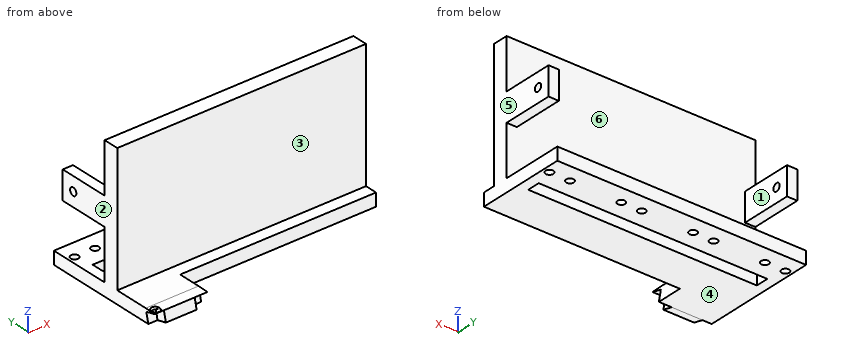
```python
from build123d import *

# Parameters (mm, degrees)
SKETCH1_W                      = 97
SKETCH1_H                      = 30
SKETCH1_R                      = 1.5
BOSS_EXTRUDE1_DEPTH            = 5
SKETCH2_W                      = 20.6
SKETCH2_H                      = 5
BOSS_EXTRUDE2_DEPTH            = 10
CUT_EXTRUDE1_REACH             = 99
CUT_EXTRUDE1_DIRECTION_2_DEPTH = 1
BOSS_EXTRUDE3_DEPTH            = 20.6
SKETCH5_W                      = 12
SKETCH5_H                      = 3.995489472
BOSS_EXTRUDE4_DEPTH            = 4.086588
SKETCH6_R                      = 1.6
CUT_EXTRUDE3_DEPTH             = 2
SKETCH7_W                      = 97
SKETCH7_H                      = 5
BOSS_EXTRUDE5_DEPTH            = 5
SKETCH8_W                      = 89.150949319
SKETCH8_H                      = 5
CUT_EXTRUDE5_DEPTH             = 6
SKETCH10_W                     = 97
SKETCH10_H                     = 6
BOSS_EXTRUDE7_DEPTH            = 50
SKETCH11_W                     = 4
SKETCH11_H                     = 11
BOSS_EXTRUDE8_DEPTH            = 20
SKETCH12_R                     = 1.5
CUT_EXTRUDE6_DEPTH             = 98


with BuildPart() as part:
    # Sketch1 → Boss-Extrude1 (new body)
    with BuildSketch(Plane.XY):
        Rectangle(SKETCH1_W, SKETCH1_H)
        with Locations((-46, 13.2)):
            Circle(SKETCH1_R, mode=Mode.SUBTRACT)
        with Locations((-38, 13.2)):
            Circle(SKETCH1_R, mode=Mode.SUBTRACT)
        with Locations((-18, 13.2)):
            Circle(SKETCH1_R, mode=Mode.SUBTRACT)
        with Locations((-10, 13.2)):
            Circle(SKETCH1_R, mode=Mode.SUBTRACT)
        with Locations((10, 13.2)):
            Circle(SKETCH1_R, mode=Mode.SUBTRACT)
        with Locations((18, 13.2)):
            Circle(SKETCH1_R, mode=Mode.SUBTRACT)
        with Locations((38, 13.2)):
            Circle(SKETCH1_R, mode=Mode.SUBTRACT)
        with Locations((46, 13.2)):
            Circle(SKETCH1_R, mode=Mode.SUBTRACT)
    extrude(amount=-BOSS_EXTRUDE1_DEPTH)

    # Sketch2 → Boss-Extrude2 (add)
    with BuildSketch(Plane.XZ.offset(15)):
        with Locations((-38.2, -2.5)):
            Rectangle(SKETCH2_W, SKETCH2_H)
    extrude(amount=BOSS_EXTRUDE2_DEPTH)

    # Sketch3 → Cut-Extrude1 (cut, up to next)
    with BuildSketch(Plane.ZY.offset(48.5), mode=Mode.PRIVATE) as cut_extrude1_sk1:
        Polygon((0, -25), (-5, -25), (0, -23.785067119), align=None)
    cut_extrude1_tool1 = extrude(cut_extrude1_sk1.sketch, amount=-CUT_EXTRUDE1_REACH, mode=Mode.PRIVATE) & part.part
    add(cut_extrude1_tool1.solids().sort_by_distance((-48.5, -24.595022, -1.666667))[0], mode=Mode.SUBTRACT)

    # Sketch3 → Cut-Extrude1 direction 2 (cut)
    with BuildSketch(Plane.ZY.offset(48.5)):
        Polygon((0, -25), (-5, -25), (0, -23.785067119), align=None)
    extrude(amount=CUT_EXTRUDE1_DIRECTION_2_DEPTH, mode=Mode.SUBTRACT)

    # Sketch4 → Boss-Extrude3 (add)
    with BuildSketch(Plane.ZY.offset(48.5)):
        Polygon((0, -23.785067119), (-1.117483581, -24.056600628), (-0.16158282, -27.990565936), align=None)
    extrude(amount=-BOSS_EXTRUDE3_DEPTH)

    # Sketch5 → Boss-Extrude4 (add)
    with BuildSketch(Plane(origin=(0, -22.459030354, 5.45724289), x_dir=(1, 0, 0), z_dir=(0, -0.971724853, 0.236116095))):
        with Locations((-38.9, -8.763781903)):
            Rectangle(SKETCH5_W, SKETCH5_H)
    extrude(amount=BOSS_EXTRUDE4_DEPTH)

    # Sketch6 → Cut-Extrude3 (cut)
    with BuildSketch(Plane(origin=(0, -1.597570275, -6.574726471), x_dir=(-1, 0, 0), z_dir=(0, -0.236116095, -0.971724853))):
        with Locations((46.634175133, -25.412540847)):
            Circle(SKETCH6_R)
    extrude(amount=-CUT_EXTRUDE3_DEPTH, mode=Mode.SUBTRACT)

    # Sketch7 → Boss-Extrude5 (add, through all)
    with BuildSketch(Plane.XY):
        with Locations((0, 17.5)):
            Rectangle(SKETCH7_W, SKETCH7_H)
    extrude(amount=-BOSS_EXTRUDE5_DEPTH)

    # Sketch8 → Cut-Extrude5 (cut, through all)
    with BuildSketch(Plane.XY):
        with Locations((-0.104637264, 3.7)):
            Rectangle(SKETCH8_W, SKETCH8_H)
    extrude(amount=-CUT_EXTRUDE5_DEPTH, mode=Mode.SUBTRACT)

    # Sketch10 → Boss-Extrude7 (add)
    with BuildSketch(Plane.XY):
        with Locations((0, -7.199863622)):
            Rectangle(SKETCH10_W, SKETCH10_H)
    extrude(amount=BOSS_EXTRUDE7_DEPTH)

    # Sketch11 → Boss-Extrude8 (add)
    with BuildSketch(Plane(origin=(0, -4.199863622, 0), x_dir=(1, 0, 0), z_dir=(0, 1, 0))):
        with Locations((46.5, -25)):
            Rectangle(SKETCH11_W, SKETCH11_H)
        with Locations((-46.5, -25)):
            Rectangle(SKETCH11_W, SKETCH11_H)
    extrude(amount=BOSS_EXTRUDE8_DEPTH)

    # Sketch12 → Cut-Extrude6 (cut, through all)
    with BuildSketch(Plane.ZY.offset(48.5)):
        with Locations((25, 10.800136378)):
            Circle(SKETCH12_R)
    extrude(amount=-CUT_EXTRUDE6_DEPTH, mode=Mode.SUBTRACT)


solid = part.part
```
Part model, mm, in its own coordinate system. Face numbers are marked on the shaded views. A direction names the side the tool comes from. Coordinates: 2 decimals unless noted, no trailing zeros. Loops run counter-clockwise (first coordinate to the right, second up) from the corner with the lowest first, then second, coordinate; pieces in that order, holes last. Notation, with made-up numbers: (40, -26.75) - (73, -26.75) arc R19 cw to (73, -13.75) - close; hole circle Ø4 at (-30, 31). An arc over 180 degrees is marked (long way). Write item = value, one per line. Start each with the question number.
Item 1: Mould opens along X. For the marked faces 4, 5 and 6 say: released by +X, released by -X, zero draft, split by the parting line, or undercut.
Item 2: Wall check: L1, parallel to Y at x = 42, z = -3; L2, parallel to Y at x = -16, z = 45.5; L3, parallel to X at y = 8.5, z = 20.5. Give the ranges that are in metal, low to high. Write a range as from..to.
Item 3: Cut at C-C, the plane z = 17. Give the cut face in (x, y).
Item 4: Cut at B-B, the plane x = -38. State how many separate pieces and enclosed holes the cut face has, and give its area (3 significant figures).
Item 5: 3-axis set-ups, long thin cutter, end or side, ignore diameter. For the marked faces 1, 2 and 3: which of +Z, -Z, +X, -X, +Y, -Y reach the whole face in a straight line?
Item 6: Flat gauge pins, fed straight in: pin 1 Ø3 at (x, y) = (47.5, 6.5) entering from +Z; pin 2 Ø4 at (x, y) = (10, 13.2) entering from +Z; pin 3 Ø3 at (x, z) = (-28, 26) entering from -Y. Where does each tip first touch, or does it go through?
Item 7: Cut at A-A, the plane x = 35.5. Give the cut face in (y, z), and give its area (3 significant figures).
The answers:
q1.face_4 = zero draft
q1.face_5 = released by +X
q1.face_6 = undercut
q2.L1 = -15..1.2, 6.2..20
q2.L2 = -10.2..-4.2
q2.L3 = -48.5..-44.5, 44.5..48.5
q3.outline = (-48.5, -10.2) - (48.5, -10.2) - (48.5, -4.2) - (-48.5, -4.2) - close
q4.separate_pieces = 3
q4.enclosed_holes = 0
q4.area = 501 mm2
q5.face_1 = +Z, +Y
q5.face_2 = +Z, -Z, -X, +Y, -Y
q5.face_3 = +Z, +X, -X, -Y
q6.pin_1 = 30.5
q6.pin_2 = 0
q6.pin_3 = -10.2
q7.outline = (-15, -5) - (1.2, -5) - (1.2, 0) - (-4.2, 0) - (-4.2, 50) - (-10.2, 50) - (-10.2, 0) - (-15, 0) - close; (6.2, -5) - (20, -5) - (20, 0) - (6.2, 0) - close
q7.area = 450 mm2
